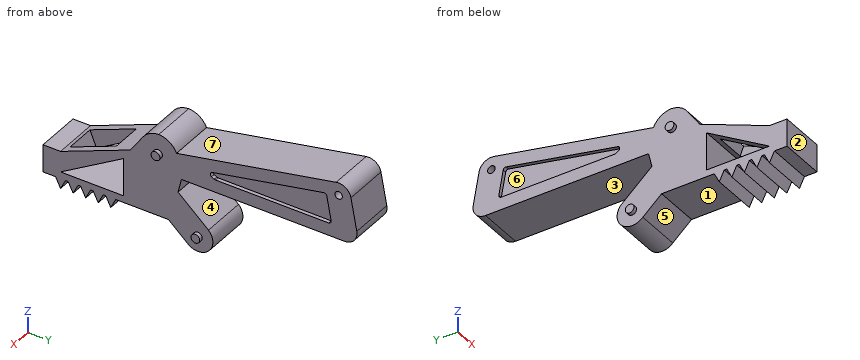
```python
from build123d import *

# Parameters (mm, degrees)
BOSS_EXTRUDE1_DEPTH = 9
CUT_EXTRUDE1_DEPTH  = 25
BOSS_EXTRUDE2_DEPTH = 18
LPATTERN1_COUNT     = 5
LPATTERN1_PITCH     = 5
FILLET1_R           = 8
FILLET2_R           = 5
SKETCH5_R           = 1.5
CUT_EXTRUDE2_DEPTH  = 25
SKETCH8_W           = 12
SKETCH8_H           = 19.929795107
CUT_EXTRUDE4_DEPTH  = 8
SKETCH9_R           = 1.75
BOSS_EXTRUDE3_DEPTH = 1.5
SKETCH10_R          = 1.75
BOSS_EXTRUDE4_DEPTH = 1.5
CUT_EXTRUDE6_DEPTH  = 1.5


with BuildPart() as part:
    # Sketch1 → Boss-Extrude1 (new, symmetric)
    with BuildSketch(Plane(origin=(0, 0, 0), x_dir=(0, 0, -1), z_dir=(1, 0, 0))):
        Polygon((55.671385575, -3.239060519), (62.288855516, 4.258211757), (53.803574142, 12.743493131), (43.094739802, 0.610903558), (37.450270875, 1.961830752), (27.646512788, -0.009546276), (22.744633745, -0.995234789), (22.744633745, -10.995234789), (33.405472618, -18.4347586), (44.671385575, -46.239060519), (44.671385575, -53.239060519), (55.671385575, -53.239060519), align=None)
        Polygon((37.450270875, 1.961830752), (27.646512788, -0.009546276), (13.846873598, 68.616760329), (37.450270875, 72.961830752), align=None)
        with BuildLine():
            ThreePointArc((62.288855516, 4.258211757), (62.288855516, 12.743493131), (53.803574142, 12.743493131))
            Line((53.803574142, 12.743493131), (62.288855516, 4.258211757))
        make_face()
    extrude(amount=BOSS_EXTRUDE1_DEPTH, both=True)

    # Sketch3 → Cut-Extrude1 (cut)
    with BuildSketch(Plane(origin=(9, 0, 0), x_dir=(0, 0, -1), z_dir=(1, 0, 0))):
        Polygon((52.971385575, -46.239060519), (52.971385575, -21.239060519), (37.971385575, -21.239060519), align=None)
    extrude(amount=-CUT_EXTRUDE1_DEPTH, mode=Mode.SUBTRACT)

    # Sketch4 → Boss-Extrude2 (add)
    with BuildSketch(Plane(origin=(9, 0, 0), x_dir=(0, 0, -1), z_dir=(1, 0, 0))):
        Polygon((55.671385575, -44.239060519), (55.671385575, -46.239060519), (59.671385575, -46.239060519), align=None)
        Polygon((59.671385575, -46.239060519), (55.671385575, -46.239060519), (55.671385575, -48.239060519), align=None)
    boss_extrude2 = extrude(amount=-BOSS_EXTRUDE2_DEPTH)

    # LPattern1: Boss-Extrude2 ×5
    with Locations(*[(0, i * LPATTERN1_PITCH, 0) for i in range(1, LPATTERN1_COUNT)]):
        add(boss_extrude2)

    # Fillet1
    # the kernel refuses this fillet: 8 mm, written as the material it takes off along each edge
    with BuildSketch(Plane(origin=(-19.431592215, -10.995234789, -22.744633745), x_dir=(0, 1, 0), z_dir=(1, 0, 0))) as fillet1_piece_1:
        with BuildLine():
            CenterArc((FILLET1_R * 0.521579610744, -FILLET1_R), FILLET1_R, 90, 55.091253842)
            Line((-FILLET1_R * 0.298484917938, -FILLET1_R * 0.427728937655), (-FILLET1_R * 0.314886208512, -FILLET1_R * 0.416283516408))
            Line((-FILLET1_R * 0.314886208512, -FILLET1_R * 0.416283516408), (-FILLET1_R * 0.0104315922149, FILLET1_R * 0.02))
            Line((-FILLET1_R * 0.0104315922149, FILLET1_R * 0.02), (FILLET1_R * 0.521579610744, FILLET1_R * 0.02))
            Line((FILLET1_R * 0.521579610744, FILLET1_R * 0.02), (FILLET1_R * 0.521579610744, 0))
        make_face()
    extrude(amount=38.86318443, mode=Mode.SUBTRACT)
    with BuildSketch(Plane(origin=(-24.975146678, -0.995234789, -22.744633745), x_dir=(0, 0.1971377027252409, -0.9803758086388171), z_dir=(1, 0, 0))) as fillet1_piece_2:
        with BuildLine():
            CenterArc((6.583284982, -7.841760559), FILLET1_R, 101.414804466, 67.215566165)
            Line((-1.259721487, -6.264658937), (-1.416581616, -6.233116905))
            Line((-1.416581616, -6.233116905), (-0.156860129, 0.031542032))
            Line((-0.156860129, 0.031542032), (0, 0.16))
            ThreePointArc((0, 0.16), (2.5, 0.16), (4.9683343, 0.156835211))
            Line((4.9683343, 0.156835211), (5, 0))
        make_face()
    extrude(amount=49.950293357, mode=Mode.SUBTRACT)

    # Fillet2
    fillet2_edges = [part.edges().sort_by_distance(p)[0] for p in [
        (0, 68.616760329, -13.846873598),
        (0, 72.961830752, -37.450270875),
    ]]
    fillet(fillet2_edges, radius=FILLET2_R)

    # Sketch5 → Cut-Extrude2 (cut)
    with BuildSketch(Plane(origin=(9, 0, 0), x_dir=(0, 0, -1), z_dir=(1, 0, 0))):
        with Locations((19.750729409, 64.619567483)):
            Circle(SKETCH5_R)
    extrude(amount=-CUT_EXTRUDE2_DEPTH, mode=Mode.SUBTRACT)

    # Sketch8 → Cut-Extrude4 (cut)
    with BuildSketch(Plane(origin=(0, 9.02689363, -22.278396507), x_dir=(1, 0, 0), z_dir=(0, -0.3755304319039708, 0.926810063990469))):
        with Locations((0, -47.762420436)):
            Rectangle(SKETCH8_W, SKETCH8_H)
    extrude(amount=-CUT_EXTRUDE4_DEPTH, mode=Mode.SUBTRACT)

    # Sketch9 → Boss-Extrude3 (add)
    with BuildSketch(Plane(origin=(9, 0, 0), x_dir=(0, 0, -1), z_dir=(1, 0, 0))):
        with Locations((58.046214829, 8.500852444)):
            Circle(SKETCH9_R)
    boss_extrude3 = extrude(amount=BOSS_EXTRUDE3_DEPTH)

    # Sketch10 → Boss-Extrude4 (add)
    with BuildSketch(Plane(origin=(9, 0, 0), x_dir=(0, 0, -1), z_dir=(1, 0, 0))):
        with Locations((30.744633745, -7.385293461)):
            Circle(SKETCH10_R)
    boss_extrude4 = extrude(amount=BOSS_EXTRUDE4_DEPTH)

    # Sketch11 → Cut-Extrude6 (cut)
    with BuildSketch(Plane(origin=(9, 0, 0), x_dir=(0, 0, -1), z_dir=(1, 0, 0))):
        with BuildLine():
            Line((32.450270875, 60.672480234), (32.450270875, 15.509128812))
            ThreePointArc((32.450270875, 15.509128812), (32.418490768, 15.259028355), (32.325170397, 15.024824336))
            Line((32.325170397, 15.024824336), (31.735253047, 13.959134396))
            ThreePointArc((31.735253047, 13.959134396), (30.707391109, 13.455206865), (29.879977716, 14.246301169))
            Line((29.879977716, 14.246301169), (20.936945668, 58.720453776))
            ThreePointArc((20.936945668, 58.720453776), (21.089259967, 59.478228738), (21.736276876, 59.901066366))
            Line((21.736276876, 59.901066366), (31.269226274, 61.655955121))
            ThreePointArc((31.269226274, 61.655955121), (32.09017532, 61.440934723), (32.450270875, 60.672480234))
        make_face()
    cut_extrude6 = extrude(amount=-CUT_EXTRUDE6_DEPTH, mode=Mode.SUBTRACT)

    # Mirror1: Boss-Extrude3, Boss-Extrude4, Cut-Extrude6 across plane
    add(boss_extrude3.mirror(Plane(origin=(0, 0, 0), x_dir=(0, 0, 1), z_dir=(1, 0, 0))))
    add(boss_extrude4.mirror(Plane(origin=(0, 0, 0), x_dir=(0, 0, 1), z_dir=(1, 0, 0))))
    add(cut_extrude6.mirror(Plane(origin=(0, 0, 0), x_dir=(0, 0, 1), z_dir=(1, 0, 0))), mode=Mode.SUBTRACT)


solid = part.part
```
Can you work these out from the model? Positions are in its coordinate system, mm. Face numbers are marked on the shaded views. A direction names the side the tool comes from. Give positions to 0.01 mm unless a question says otherwise; leave off trailing zeros. Write each loop counter-clockwise with the first axis right and the second up, starting at its lowest first coordinate (ties: lowest second). Pieces come first, ordered by that corner, then holes. Notation, with made-up numbers: (86.25, -36) - (118.25, -36) arc R17 cw to (118.25, -10) - close; hole circle Ø10 at (83, 27.5). An arc over 180 degrees is marked (long way). Write item = value, one per line. Start each with the question number.
1. Imagine slicing it at C-C (y = 42.5). Please give me the cut outline in (x, z), and give its area (3 significant figures).
2. For pin 1 (5 mm diameter, centred on x = 5, y = -5.5, fed in from +Z); pin 2 (1 mm diameter, centred on x = -2, z = -35.5, fed in from -Y); pin 3 (9 mm diameter, centred on y = 27.5, z = -24, fed in from -X), each with a flat end and sliding along its axis, tell me the tip position at first contact or that it passes through.
3. Thinking about a two-plate mould opening in Y: for the marked faces 1, 2 and 3, which applies, released by +Y, released by -Y, zero draft, split by the parting line, or undercut?
4. Please list where these lines run through material, in increasing order: line 1 (Y direction, x = 6.5, z = -41); line 2 (Y direction, x = 4.5, z = -50); line 3 (X direction, y = 3, z = -49).
5. Imagine slicing it at B-B (z = -47). Please give me the cut outline in (x, y).
6. Imagine slicing it at A-A (z = -58). Count the separate pieces of the cut face and the enclosed holes in it, and give its area (3 significant figures).
7. On a 3-axis mill with a long thin cutter (end or side, diameter ignored), from which of +Z, -Z, +X, -X, +Y, -Y can I reach the whole of each face in a straight line? I mean the marked faces 4, 5, 6 and 7. Say none if no direction works.
Worked answers:
q1.outline = (-9, -37.45) - (9, -37.45) - (9, -32.45) - (7.5, -32.45) - (7.5, -24.2) - (9, -24.2) - (9, -19.1) - (-9, -19.1) - (-9, -24.2) - (-7.5, -24.2) - (-7.5, -32.45) - (-9, -32.45) - close
q1.area = 306 mm2
q2.pin_1 = -22.75
q2.pin_2 = -24.84
q2.pin_3 = -9
q3.face_1 = undercut
q3.face_2 = released by -Y
q3.face_3 = zero draft
q4.line_1 = -37.18 to -26.29, -21.24 to 1.11
q4.line_2 = -53.24 to -42.03, -21.24 to 8.43
q4.line_3 = -9 to 9
q5.outline = (-9, -53.24) - (9, -53.24) - (9, -36.29) - (6, -36.29) - (6, -43.24) - (-6, -43.24) - (-6, -36.29) - (-9, -36.29) - close; (-9, -21.24) - (9, -21.24) - (9, 5.04) - (-9, 5.04) - close
q6.separate_pieces = 6
q6.enclosed_holes = 0
q6.area = 433 mm2
q7.face_4 = +X, -X, +Y
q7.face_5 = -Z, +X, -X
q7.face_6 = -X
q7.face_7 = +Z, +X, -X
